Design review of the part shown in the three views and the two pictorial views. Dimensions are in mm from the part's minimum x, y and z. A direction names the side the tool comes from. Coordinates: 2 decimals unless noted, no trailing zeros. Loops run counter-clockwise (first coordinate to the right, second up) from the corner with the lowest first, then second, coordinate; pieces in that order, holes last. Notation, with made-up numbers: (70.5, -5.5) -> (84.5, -5.5) arc R19 ccw to (84.5, 15.5) -> close; hole circle Ø1 at (81.25, 55.5). An arc over 180 degrees is marked (long way). Answer in a Markdown table with one row per item.
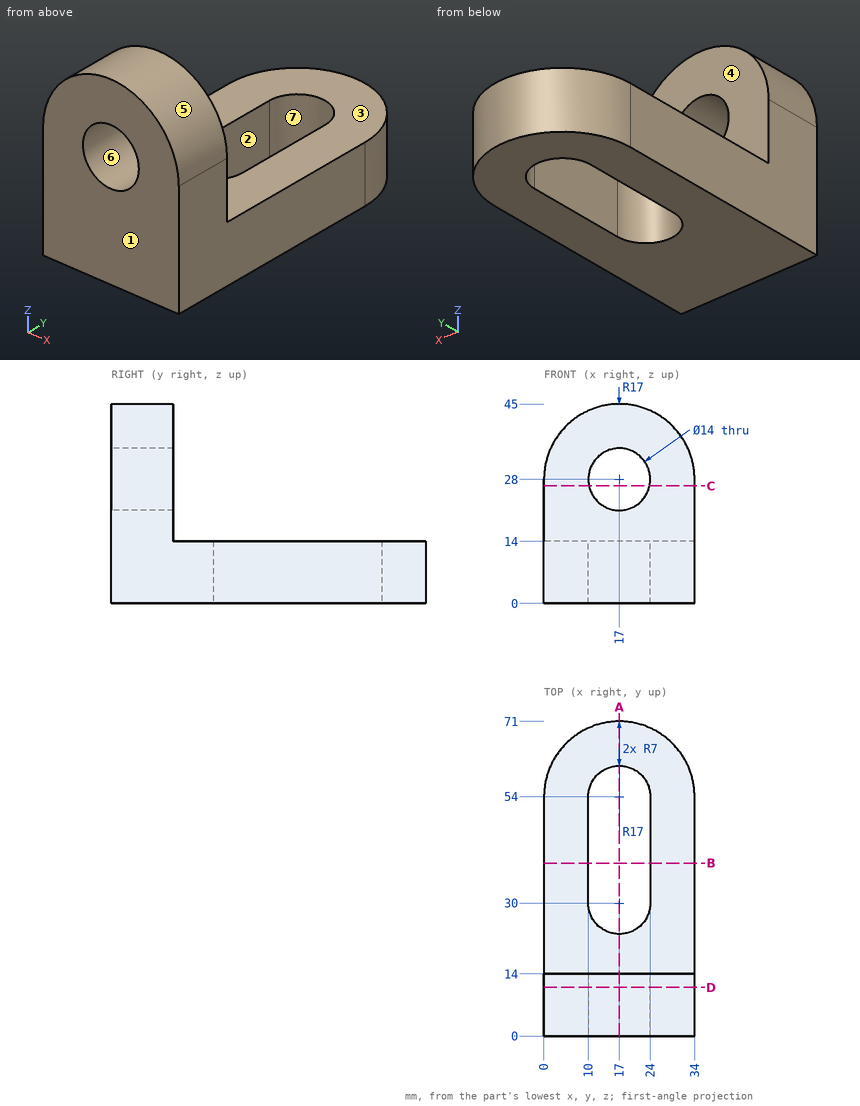
Item 1: Take a section at B-B, the plane y = 39. State the section outline as (x, z) points, and give its area (3 significant figures).
Worked answers:
| item | result |
|---|---|
| outline | (0, 0) -> (10, 0) -> (10, 14) -> (0, 14) -> close; (24, 0) -> (34, 0) -> (34, 14) -> (24, 14) -> close |
| area | 280 mm² |
Item 2: Insertion check: pin 1 (3 mm diameter, centred on x = 18, z = 11.5, fed in from -Y); pin 2 (4 mm diameter, centred on x = 4.5, y = 60, fed in from +Z); pin 3 (11 mm diameter, centred on x = 17, z = 28, fed in from -Y). Each pin has a flat end and moves straight along its axis. Give the tip position at first contact, or say it passes through.
Worked answers:
| item | result |
|---|---|
| pin 1 | y = 0 |
| pin 2 | z = 14 |
| pin 3 | through |
Item 3: Take a section at A-A, the plane x = 17. State the section outline as (y, z) points, and give its area (3 significant figures).
Worked answers:
| item | result |
|---|---|
| outline | (0, 0) -> (23, 0) -> (23, 14) -> (14, 14) -> (14, 21) -> (0, 21) -> close; (0, 35) -> (14, 35) -> (14, 45) -> (0, 45) -> close; (61, 0) -> (71, 0) -> (71, 14) -> (61, 14) -> close |
| area | 700 mm² |
Item 4: The part is to be moulded in two halves that separate along X. For the marked faces 4, 5, 6 and 7, say which applies: +X half, -X half, draft (parallel to the pull), parting line (faces both ways), or undercut.
Worked answers:
| item | result |
|---|---|
| face 4 | draft |
| face 5 | parting line |
| face 6 | undercut |
| face 7 | undercut |
Item 5: Take a section at D-D, the plane y = 11. State the section outline as (x, z) points.
Worked answers:
| item | result |
|---|---|
| outline | (0, 0) -> (34, 0) -> (34, 28) arc R17 ccw to (0, 28) -> close; hole circle Ø14 at (17, 28) |
Item 6: For L1, parallel to X at y = 42.5, z = 4; L2, parallel to Z at x = 17, y = 11; L3, parallel to Z at x = 33.5, y = 45, list the stretches that pass through material, from the lowest coordinate up.
Worked answers:
| item | result |
|---|---|
| L1 | 0 to 10, 24 to 34 |
| L2 | 0 to 21, 35 to 45 |
| L3 | 0 to 14 |
Item 7: For the marked faces 1, 2 and 3, list the 3-axis set-ups (+Z, -Z, +X, -X, +Y, -Y) from which the entire face can be reached by the end or side of a thin tool; tool diameter is ignored.
Worked answers:
| item | result |
|---|---|
| face 1 | +Z, -Z, +X, -X, -Y |
| face 2 | +Z, -Z |
| face 3 | +Z, +X, -X, +Y |
Item 8: Take a section at C-C, the plane z = 26.5. State the section outline as (x, y) points.
Worked answers:
| item | result |
|---|---|
| outline | (0, 0) -> (10.16, 0) -> (10.16, 14) -> (0, 14) -> close; (23.84, 0) -> (34, 0) -> (34, 14) -> (23.84, 14) -> close |
